Build history of the part. All positions in model axes, mm. A direction names the side the tool comes from. Give positions to 0.01 mm unless a question says otherwise; leave off trailing zeros. Loops run counter-clockwise (first coordinate to the right, second up) from the corner with the lowest first, then second, coordinate; pieces in that order, holes last.
1) Band-saw the part on C-C on x = -13.85. List the corners of the cut face in (y, z).
2) Band-saw the part on A-A on x = -37. List the corners of the cut face in (y, z), then the cut area to 3 significant figures.
3) 3-axis set-ups, long thin cutter, end or side, ignore diameter. For faces 1 (the flat face through (4, 8.5, -10)), 2 (the flat face through (-45, -13.5, -8)), 3 (the flat face through (-14, 0, -23)): which of +Z, -Z, +X, -X, +Y, -Y reach the whole face in a straight line?
4) Wall check: line 1 (X direction, y = -4.5, z = -10.25); line 2 (X direction, y = 7.6, z = -21.25); line 3 (Z direction, x = -16.5, y = 4). Give the ranges that are in metal, low to high.
5) Two-plate mould, pull along Z, no slides. Class faces 4 (the flat face through (3.2, 8, -21)), 5 (the flat face through (7, -7, -19.5)), 6 (the cylindrical face through (-10.02, 9.07, -4.4)), 7 (the flat face through (-68.4, 15, -10)): +Z half, -Z half, draft (parallel to the pull), parting line (faces both ways), or undercut.
6) Flat gauge pins, fed straight in: P1, Ø5, axis at x = -27, z = -10.5, coming from the +Y side; P2, Ø1.4, axis at x = -14.5, y = 0, coming from the +Z side; P3, Ø1.8, axis at x = -22, y = -13, coming from the +Z side; P4, Ø5, axis at x = -13, z = 1, coming from the -Y side. Where does each tip first touch, or does it go through?
7) Band-saw the part on B-B on z = -10.25. State how many separate pieces and enclosed holes the cut face has, then the cut area to 3 significant figures.
```python
from build123d import *

# Parameters (mm, degrees)
SKETCH1_R                = 1.4
BOSS_EXTRUDE1_DEPTH      = 2
BOSS_EXTRUDE1_2_DEPTH    = 2
BOSS_EXTRUDE3_DEPTH      = 2.5
BOSS_EXTRUDE3_DEPTH_BACK = 25
SKETCH4_W                = 36.8
SKETCH4_H                = 17
BOSS_EXTRUDE4_START      = 23
SKETCH5_W                = 4.7
SKETCH5_H                = 13
SKETCH5_R                = 1.4
BOSS_EXTRUDE4_DEPTH      = 23
SKETCH6_W                = 36.8
SKETCH6_H                = 17
BOSS_EXTRUDE5_DEPTH      = 2
SKETCH7_R                = 1.5
SKETCH7_W                = 8.5
SKETCH7_H                = 3.5
CUT_EXTRUDE1_DEPTH       = 36.391524409
SKETCH8_R                = 1.5
CUT_EXTRUDE2_DEPTH       = 46.293376999
CUT_EXTRUDE3_DEPTH       = 36.791898525
BOSS_EXTRUDE6_DEPTH      = 10
CUT_EXTRUDE4_DEPTH       = 79.762681519
CUT_EXTRUDE4_DEPTH_BACK  = 79.762681519
FILLET1_R                = 2


with BuildPart() as part:
    # Sketch1 → Boss-Extrude1 (new body)
    with BuildSketch(Plane.XY):
        Polygon((-11.7, -6.5), (-11.7, 0), (-11.7, 6.5), (-16.4, 6.5), (-16.4, -6.5), align=None)
        with Locations((-13.85, 0)):
            Circle(SKETCH1_R, mode=Mode.SUBTRACT)
    extrude(amount=BOSS_EXTRUDE1_DEPTH)



with BuildPart() as body_2:
    # Sketch1 → Boss-Extrude1 2 (new body)
    with BuildSketch(Plane.XY):
        Polygon((11.7, 6.5), (11.7, 0), (11.7, -6.5), (16.4, -6.5), (16.4, 6.5), align=None)
        with Locations((13.85, 0)):
            Circle(SKETCH1_R, mode=Mode.SUBTRACT)
    extrude(amount=BOSS_EXTRUDE1_2_DEPTH)


with BuildPart() as part_1:
    add(part.part)

    add(body_2.part)  # Boss-Extrude3 merges body 2
    # Sketch4 → Boss-Extrude3 (add, two sides: drawn at the far end of the back side and taken through both)
    with BuildSketch(Plane.XY.offset(2).offset(-BOSS_EXTRUDE3_DEPTH_BACK)):
        Rectangle(SKETCH4_W, SKETCH4_H)
        Polygon((-16.4, 6.5), (-11.7, 6.5), (11.7, 6.5), (16.4, 6.5), (16.4, -6.5), (11.7, -6.5), (-11.7, -6.5), (-16.4, -6.5), align=None, mode=Mode.SUBTRACT)
    extrude(amount=BOSS_EXTRUDE3_DEPTH + BOSS_EXTRUDE3_DEPTH_BACK)

    # Sketch5 → Boss-Extrude4 (add)
    # profile 1 of 2: a face of its own
    with BuildSketch(Plane(origin=(0, 0, 0), x_dir=(-1, 0, 0), z_dir=(0, 0, -1)).offset(BOSS_EXTRUDE4_START)):
        with Locations((-14.05, 0)):
            Rectangle(SKETCH5_W, SKETCH5_H)
        with Locations(Location((-13.85, 0, 0), (0, 0, 180))):
            Circle(SKETCH5_R, mode=Mode.SUBTRACT)
    # profile 2 of 2: a face of its own
    with BuildSketch(Plane(origin=(0, 0, 0), x_dir=(-1, 0, 0), z_dir=(0, 0, -1)).offset(BOSS_EXTRUDE4_START)):
        with Locations((14.05, 0)):
            Rectangle(SKETCH5_W, SKETCH5_H)
        with Locations(Location((13.85, 0, 0), (0, 0, 180))):
            Circle(SKETCH5_R, mode=Mode.SUBTRACT)
    extrude(amount=-BOSS_EXTRUDE4_DEPTH)

    # Sketch6 → Boss-Extrude5 (add)
    with BuildSketch(Plane(origin=(0, 0, -23), x_dir=(-1, 0, 0), z_dir=(0, 0, -1))):
        Rectangle(SKETCH6_W, SKETCH6_H)
    extrude(amount=BOSS_EXTRUDE5_DEPTH)

    # Sketch7 → Cut-Extrude1 (cut, through all)
    with BuildSketch(Plane(origin=(0, 8.5, 0), x_dir=(1, 0, 0), z_dir=(0, 1, 0))):
        with Locations(Location((-1.300147184, 21.25, 0), (0, 0, 270))):
            Circle(SKETCH7_R)
        with Locations(Location((-9.300147184, 21.25, 0), (0, 0, 270))):
            Circle(SKETCH7_R)
        with Locations((7.45, 21.25)):
            Rectangle(SKETCH7_W, SKETCH7_H)
    extrude(amount=-CUT_EXTRUDE1_DEPTH, mode=Mode.SUBTRACT)

    # Sketch8 → Cut-Extrude2 (cut, through all)
    with BuildSketch(Plane(origin=(18.4, 0, 0), x_dir=(0, 0, -1), z_dir=(1, 0, 0))):
        with Locations(Location((20.5, 4, 0), (0, 0, 90))):
            Circle(SKETCH8_R)
        with Locations((20.5, -4)):
            Circle(SKETCH8_R)
    extrude(amount=-CUT_EXTRUDE2_DEPTH, mode=Mode.SUBTRACT)

    # Sketch9 → Cut-Extrude3 (cut, through all)
    with BuildSketch(Plane(origin=(0, 0, -25), x_dir=(-1, 0, 0), z_dir=(0, 0, -1))):
        with BuildLine():
            Line((8.9, -1.5), (-8.9, -1.5))
            ThreePointArc((-8.9, -1.5), (-10.4, 0), (-8.9, 1.5))
            Line((-8.9, 1.5), (8.9, 1.5))
            ThreePointArc((8.9, 1.5), (10.4, 0), (8.9, -1.5))
        make_face()
    extrude(amount=-CUT_EXTRUDE3_DEPTH, mode=Mode.SUBTRACT)

    # Sketch10 → Boss-Extrude6 (add)
    with BuildSketch(Plane(origin=(0, 0, -15), x_dir=(-1, 0, 0), z_dir=(0, 0, -1))):
        Polygon((68.4, -13.5), (18.4, -13.5), (18.4, -8.5), (3.4, -8.5), (3.4, -16.5), (68.4, -16.5), align=None)
        Polygon((3.4, 8.5), (18.4, 8.5), (18.4, 13.5), (68.4, 13.5), (68.4, 16.5), (3.4, 16.5), align=None)
    extrude(amount=-BOSS_EXTRUDE6_DEPTH)

    # Sketch12 → Cut-Extrude4 (cut, two sides: drawn at the far end of the back side and taken through both)
    with BuildSketch(Plane(origin=(0, -13.5, 0), x_dir=(1, 0, 0), z_dir=(0, 1, 0)).offset(-CUT_EXTRUDE4_DEPTH_BACK)):
        with BuildLine():
            Line((-24.9, 8.5), (-61.9, 8.5))
            ThreePointArc((-61.9, 8.5), (-63.4, 10), (-61.9, 11.5))
            Line((-61.9, 11.5), (-24.9, 11.5))
            ThreePointArc((-24.9, 11.5), (-23.4, 10), (-24.9, 8.5))
        make_face()
    extrude(amount=CUT_EXTRUDE4_DEPTH + CUT_EXTRUDE4_DEPTH_BACK, mode=Mode.SUBTRACT)

    # Fillet1
    fillet1_edges = [part_1.edges().sort_by_distance(p)[0] for p in [
        (-3.4, 8.5, -10),
        (-18.4, 13.5, -10),
        (-10.9, 8.5, -5),
        (-10.9, 8.5, -15),
        (-10.9, -8.5, -15),
        (-3.4, -8.5, -10),
        (-10.9, -8.5, -5),
        (-18.4, -13.5, -10),
    ]]
    fillet(fillet1_edges, radius=FILLET1_R)


solid = part_1.part
```
Findings below:
1. outline: (-16.5, -15) - (-10.5, -15) arc R2 cw to (-8.5, -17) - (-8.5, -25) - (8.5, -25) - (8.5, -17) arc R2 cw to (10.5, -15) - (16.5, -15) - (16.5, -5) - (10.5, -5) arc R2 cw to (8.5, -3) - (8.5, 4.5) - (6.5, 4.5) - (6.5, 2) - (1.4, 2) - (1.4, -23) - (-1.4, -23) - (-1.4, 2) - (-6.5, 2) - (-6.5, 4.5) - (-8.5, 4.5) - (-8.5, -3) arc R2 cw to (-10.5, -5) - (-16.5, -5) - close; hole circle Ø3 at (-4, -20.5); hole circle Ø3 at (4, -20.5)
2. outline: (-16.5, -15) - (-13.5, -15) - (-13.5, -11.5) - (-16.5, -11.5) - close; (-16.5, -8.5) - (-13.5, -8.5) - (-13.5, -5) - (-16.5, -5) - close; (13.5, -15) - (16.5, -15) - (16.5, -11.5) - (13.5, -11.5) - close; (13.5, -8.5) - (16.5, -8.5) - (16.5, -5) - (13.5, -5) - close
2. area: 42.0 mm2
3. face 1: +X, +Y
3. face 2: +Z, -Z, -X
3. face 3: +Z
4. line 1: x = -18.4 to -11.7, 11.7 to 18.4
4. line 2: x = -18.4 to -10.8, -7.8 to -2.8, 0.2 to 3.2, 11.7 to 18.4
4. line 3: z = -25 to -22, -19 to 4.5
5. face 4: undercut
5. face 5: undercut
5. face 6: +Z half
5. face 7: draft
6. P1: stops at y = 16.5
6. P2: stops at z = -23
6. P3: stops at z = -5
6. P4: stops at y = -8.5
7. separate pieces: 3
7. enclosed holes: 3
7. area: 613 mm2
